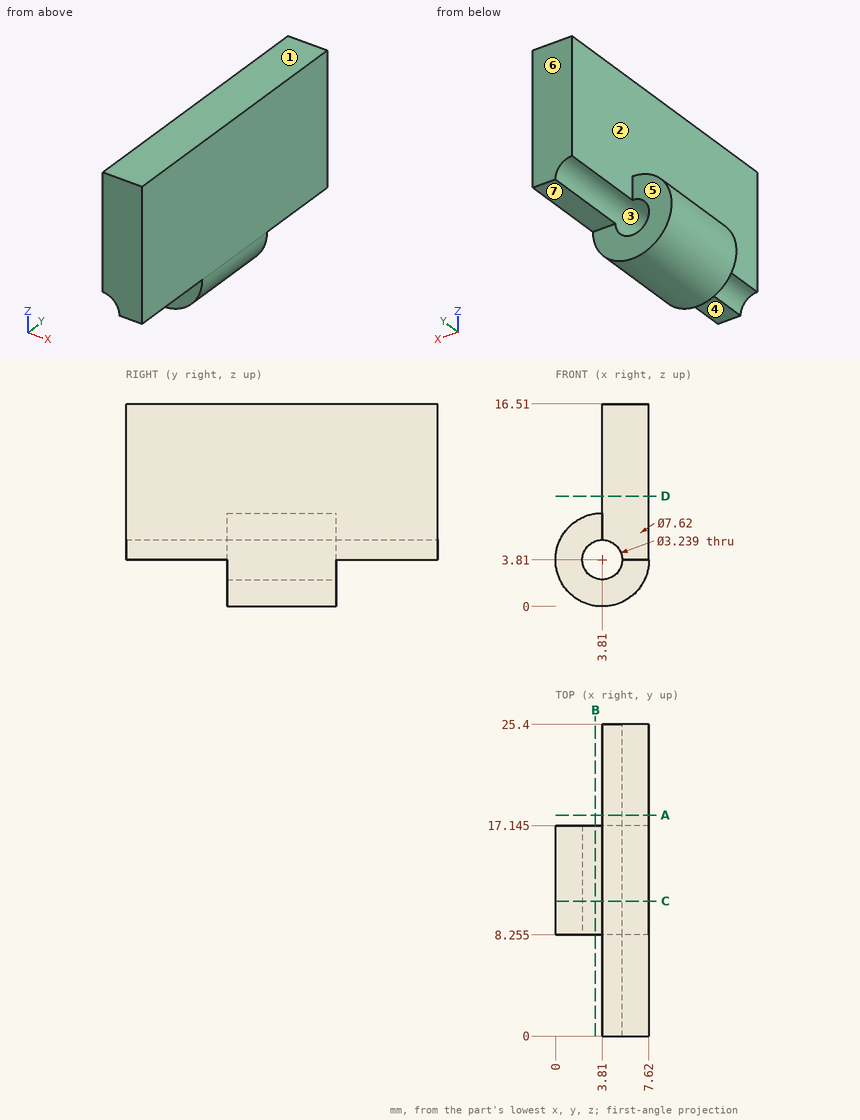
Answer from the drawing. Dimensions are ordinates in mm from the lowest x, y and z of the part. A direction names the side the tool comes from. Give positions to 0.01 mm unless a question says otherwise; leave off trailing zeros. Order: outer loops, then holes, each group sorted by start corner. A loop starts at its lowest first (then second) coordinate and runs counter-clockwise, first axis right, second up. Notation, with made-up numbers: (46.25, 11.25) -> (99.25, 11.25) arc R17 cw to (99.25, 34.25) -> close; hole circle Ø5 at (17, 25). An arc over 180 degrees is marked (long way). One line per item, written item: value. Start each with the question number.
(1) The part is cut by section B-B (x = 3.25). Determine the outline of the cut face in (y, z) (1 decimal).
(2) The part is cut by section A-A (y = 18). Determine the outline of the cut face in (x, z).
(3) For a pull along Z with two mould halves and no side action, classify the marked faces 1, 2, 3 and 4 as released by +Z, released by -Z, zero draft, split by the parting line, or undercut.
(4) Flat-ended cylindrical pins translate along their axes: P1, Ø1.5, axis at y = 22, z = 5.5, coming from the -X side; P2, Ø2, axis at x = 1, z = 3.5, coming from the -Y side (1 decimal); P3, Ø2.5, axis at x = 6.5, y = 22.5, coming from the -Z side. Find the tip coordinate at first contact, or state that the pin passes through.
(5) The part is cut by section D-D (z = 9). Determine the outline of the cut face in (x, y).
(6) Straight lines are drawn through the part: L1, parallel to X at y = 13, z = 3.75; L2, parallel to Y at x = 1, z = 4.75 (1 decimal); L3, parallel to X at y = 5.25, z = 15.5. For each, find the intervals that lie inside material, in ascending order.
(7) The part is cut by section C-C (y = 11). Determine the outline of the cut face in (x, z).
(8) A tool of negligible diameter and unlimited length cuts with its end or side. For the marked faces 5, 6 and 7, from which of +Z, -Z, +X, -X, +Y, -Y can it reach the whole face along a straight path? Write none if from no direction.
Taken from the geometry:
1. outline: (8.3, 0) -> (17.1, 0) -> (17.1, 2.3) -> (8.3, 2.3) -> close; (8.3, 5.3) -> (17.1, 5.3) -> (17.1, 7.6) -> (8.3, 7.6) -> close
2. outline: (3.81, 5.43) arc R1.62 cw to (5.43, 3.81) -> (7.62, 3.81) -> (7.62, 16.51) -> (3.81, 16.51) -> close
3. face 1: released by +Z
3. face 2: zero draft
3. face 3: undercut
3. face 4: released by -Z
4. P1: x = 3.81
4. P2: y = 8.3
4. P3: z = 3.81
5. outline: (3.81, 0) -> (7.62, 0) -> (7.62, 25.4) -> (3.81, 25.4) -> close
6. L1: 0 to 2.19, 5.43 to 7.62
6. L2: 8.3 to 17.1
6. L3: 3.81 to 7.62
7. outline: (3.81, 7.62) arc R3.81 ccw (long way) to (7.62, 3.81) -> (7.62, 16.51) -> (3.81, 16.51) -> close; hole circle Ø3.24 at (3.81, 3.81)
8. face 5: -Z, -X, +Y
8. face 6: +Z, -Z, +X, -X, +Y
8. face 7: -Z, +X, -X, +Y
